```python
from build123d import *

# Parameters (mm, degrees)
SALIENTE_EXTRUIR1_DEPTH = 100
SALIENTE_EXTRUIR2_DEPTH = 6
CROQUIS4_R              = 1.5
CROQUIS4_W              = 80
CROQUIS4_H              = 60
CORTAR_EXTRUIR2_DEPTH   = 6
CROQUIS5_R              = 2.6
CORTAR_EXTRUIR3_DEPTH   = 358.888250715


with BuildPart() as part:
    # Croquis1 → Saliente-Extruir1 (new body)
    with BuildSketch(Plane.XY):
        Polygon((-41, 72), (-161, 72), (-161, -70), (-41, -70), (-41, -120), (41, -120), (41, -70), (161, -70), (161, 72), (41, 72), (41, 120), (-41, 120), align=None)
        Polygon((155, 66), (35, 66), (35, 114), (-35, 114), (-35, 66), (-155, 66), (-155, -64), (-35, -64), (-35, -114), (35, -114), (35, -64), (155, -64), align=None, mode=Mode.SUBTRACT)
    extrude(amount=SALIENTE_EXTRUIR1_DEPTH)

    # Croquis2 → Saliente-Extruir2 (add)
    with BuildSketch(Plane(origin=(0, 0, 0), x_dir=(-1, 0, 0), z_dir=(0, 0, -1))):
        Polygon((41, 72), (41, 120), (-41, 120), (-41, 72), (-161, 72), (-161, -70), (-41, -70), (-41, -120), (41, -120), (41, -70), (161, -70), (161, 72), align=None)
    extrude(amount=-SALIENTE_EXTRUIR2_DEPTH)

    # Croquis4 → Cortar-Extruir2 (cut)
    with BuildSketch(Plane(origin=(0, 72, 0), x_dir=(1, 0, 0), z_dir=(0, 1, 0))):
        with Locations(Location((151, -90, 0), (0, 0, 270))):
            Circle(CROQUIS4_R)
        with Locations(Location((51, -90, 0), (0, 0, 270))):
            Circle(CROQUIS4_R)
        with Locations(Location((51, -10, 0), (0, 0, 270))):
            Circle(CROQUIS4_R)
        with Locations(Location((151, -10, 0), (0, 0, 270))):
            Circle(CROQUIS4_R)
        with Locations((101, -50)):
            Rectangle(CROQUIS4_W, CROQUIS4_H)
    extrude(amount=-CORTAR_EXTRUIR2_DEPTH, mode=Mode.SUBTRACT)

    # Croquis5 → Cortar-Extruir3 (cut, through all)
    with BuildSketch(Plane(origin=(161, 0, 0), x_dir=(0, 0, -1), z_dir=(1, 0, 0))):
        with Locations((-60, -13.75)):
            Circle(CROQUIS5_R)
        with Locations((-60, 15.75)):
            Circle(CROQUIS5_R)
    extrude(amount=-CORTAR_EXTRUIR3_DEPTH, mode=Mode.SUBTRACT)


solid = part.part
```
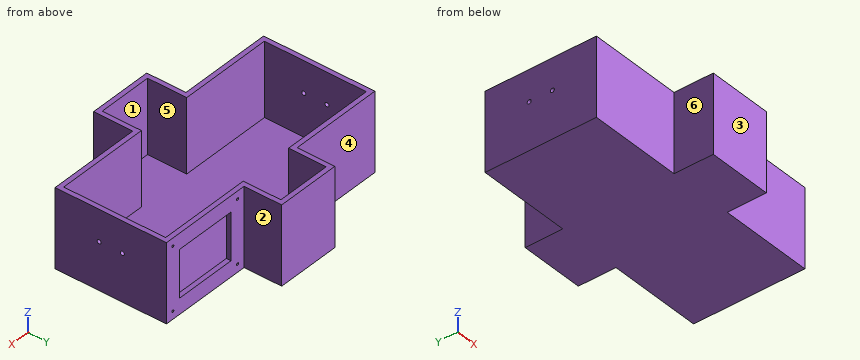
For this review, take the finished solid that the model builds, in its own axes (mm). Face numbers are marked on the shaded views. A direction names the side the tool comes from. Coordinates: 2 decimals unless noted, no trailing zeros. Write each loop counter-clockwise with the first axis right and the second up, starting at its lowest first coordinate (ties: lowest second). Pieces come first, ordered by that corner, then holes.
(1) Add section D-D on x = -64. Give the boundary of the cut face in (y, z).
(2) The part is to be moulded in two halves that separate along X. For the marked faces 1, 2 and 3, say which applies: +X half, -X half, draft (parallel to the pull), parting line (faces both ways), or undercut.
(3) Add section A-A on x = 87. Give the boundary of the cut face in (y, z), then the cut area to 3 significant figures.
(4) Add section C-C on y = 44. Give the boundary of the cut face in (x, z).
(5) For pin 1 Ø2 at (y, z) = (95, 52) entering from +X; pin 2 Ø24 at (y, z) = (89, 58) entering from -X; pin 3 Ø4 at (x, y) = (102.5, 3) entering from +Z; pin 4 Ø3 at (y, z) = (15.75, 60) entering from -X, all flat-tipped, find the tip position at first contact; note any pin that passes through.
(6) Wall thickness on probe 1 along Y at (x, z) = (-158, 60); probe 2 along X at (y, z) = (68.5, 70); probe 3 along Y at (x, z) = (-118.5, 74): over which ranges is each line inside the solid? List them lowest first.
(7) Tool access review of the marked faces 4, 5 and 6: name each direction out of +Z, -Z, +X, -X, +Y, -Y from which nothing blocks a thin tool from reaching the whole face with its end or side.
(8) Add section B-B on z = 51. Give the boundary of the cut face in (x, y), then the cut area to 3 significant figures.
Answer sheet:
1. outline: (-70, 0) - (72, 0) - (72, 100) - (66, 100) - (66, 6) - (-64, 6) - (-64, 100) - (-70, 100) - close
2. face 1: undercut
2. face 2: +X half
2. face 3: draft
3. outline: (-70, 0) - (72, 0) - (72, 20) - (66, 20) - (66, 6) - (-64, 6) - (-64, 100) - (-70, 100) - close; (66, 80) - (72, 80) - (72, 100) - (66, 100) - close
3. area: 1,620 mm2
4. outline: (-161, 0) - (161, 0) - (161, 100) - (155, 100) - (155, 6) - (-155, 6) - (-155, 100) - (-161, 100) - close
5. pin 1: stops at x = 41
5. pin 2: stops at x = -41
5. pin 3: stops at z = 6
5. pin 4: passes through
6. probe 1: y = -70 to -16.35, -11.15 to 13.15, 18.35 to 72
6. probe 2: x = -161 to -35, 35 to 61, 141 to 161
6. probe 3: y = -70 to -64, 66 to 72
7. face 4: +Z, -Z, -X, +Y
7. face 5: +Z
7. face 6: +Z, -Z, -X, -Y
8. outline: (-161, -70) - (-41, -70) - (-41, -120) - (41, -120) - (41, -70) - (161, -70) - (161, 72) - (141, 72) - (141, 66) - (155, 66) - (155, -64) - (35, -64) - (35, -114) - (-35, -114) - (-35, -64) - (-155, -64) - (-155, 66) - (-35, 66) - (-35, 114) - (35, 114) - (35, 66) - (61, 66) - (61, 72) - (41, 72) - (41, 120) - (-41, 120) - (-41, 72) - (-161, 72) - close
8. area: 6,120 mm2
